Read the model definition and answer for the solid it produces. Units are mm, in the model's axes. A direction names the side the tool comes from. Coordinates: 2 decimals unless noted, no trailing zeros. Write each loop counter-clockwise with the first axis right and the second up, starting at its lowest first coordinate (ties: lowest second). Pieces come first, ordered by that corner, then holes. Notation, with made-up numbers: (86, -5) -> (90, -5) arc R11 ccw to (90, 6) -> close; hole circle Ø7 at (58.5, 63.25). An arc over 180 degrees is marked (long way). Answer in a Markdown table with one row per item. Add a question column.
Item 1: Section B-B on x = 1.25 is taken. Write down the section's boundary in (y, z).
Item 2: Which of the six approach directions +Z, -Z, +X, -X, +Y, -Y give full straight-line access (tool end or side, diameter ignored) to faces 4 (the face through (1, 50, 35.286)), 5 (the face through (-11.25, 22, 6)), 6 (the face through (32.196, -1.479, -2.614)), 7 (the face through (1, 35, 38.286))?
Item 3: Section C-C on y = 48 is taken. Write down the section's boundary in (x, z), then the cut area to 3 significant figures.
Item 4: Given pin 1 Ø10 at (x, y) = (-9, 35) entering from +Z; pin 2 Ø1.5 at (x, z) = (-19.5, 53) entering from +Y; pin 3 Ø12 at (x, z) = (29, 13.5) entering from -Y, each flat-ended and moving along its own axis, determine where each tip first touches the part or whether it passes through.
Item 5: Section D-D on x = 15 is taken. Write down the section's boundary in (y, z), then the cut area to 3 significant figures.
Item 6: Straight lines are drawn through the part: line 1 (Y direction, x = 37, z = 50); line 2 (X direction, y = 31, z = 19.5); line 3 (Y direction, x = 9, z = 26). For each, find the intervals that lie inside material, in ascending order. Write a range as from..to.
Item 7: For a pull along X with two mould halves and no side action, classify faces 1 (the face through (-48.75, 3, 25)), 2 (the face through (-5.8, 19.27, -4.12)), 3 (the face through (13.75, 22, 7)) as +X half, -X half, draft (parallel to the pull), parting line (faces both ways), or undercut.
Item 8: Section A-A on z = 27.5 is taken. Write down the section's boundary in (x, y).
```python
from build123d import *

# Parameters (mm, degrees)
SKETCH1_W           = 100
SKETCH1_H           = 100
BOSS_EXTRUDE1_DEPTH = 38
SKETCH3_R           = 3
BOSS_EXTRUDE2_DEPTH = 3
SKETCH4_R           = 8.25
SKETCH5_R           = 9.5
SKETCH6_W           = 25
SKETCH6_H           = 3
BOSS_EXTRUDE3_DEPTH = 25
CUT_EXTRUDE3_DEPTH  = 32


with BuildPart() as part:
    # Sketch1 → Boss-Extrude1 (new body)
    with BuildSketch(Plane(origin=(0, 0, 0), x_dir=(1, 0, 0), z_dir=(0, 1, 0))):
        with Locations((1.25, -24.285714286)):
            Rectangle(SKETCH1_W, SKETCH1_H)
    extrude(amount=BOSS_EXTRUDE1_DEPTH)

    # Sketch3 → Boss-Extrude2 (add)
    with BuildSketch(Plane.XZ):
        with Locations(Location((-27.034271247, 52.569985533, 0), (0, 0, 90))):
            Circle(SKETCH3_R)
        with Locations(Location((29.534271247, 52.569985533, 0), (0, 0, 90))):
            Circle(SKETCH3_R)
        with Locations(Location((29.534271247, -3.998556962, 0), (0, 0, 90))):
            Circle(SKETCH3_R)
        with Locations(Location((-27.034271247, -3.998556962, 0), (0, 0, 90))):
            Circle(SKETCH3_R)
    extrude(amount=BOSS_EXTRUDE2_DEPTH)

    # Sketch4 → Cut-Loft1 section 0
    with BuildSketch(Plane.XZ):
        with Locations((1.25, 1.285714286)):
            Circle(SKETCH4_R)
    # Sketch5 → Cut-Loft1 section 1
    with BuildSketch(Plane(origin=(0, 38, 0), x_dir=(1, 0, 0), z_dir=(0, 1, 0))):
        with Locations((1.25, -1.285714286)):
            Circle(SKETCH5_R)
    loft(mode=Mode.SUBTRACT)

    # Sketch6 → Boss-Extrude3 (add)
    with BuildSketch(Plane(origin=(0, 38, 0), x_dir=(1, 0, 0), z_dir=(0, 1, 0))):
        with Locations((1.25, -36.785714286)):
            Rectangle(SKETCH6_W, SKETCH6_H)
    extrude(amount=BOSS_EXTRUDE3_DEPTH)

    # Sketch9 → Cut-Extrude3 (cut)
    with BuildSketch(Plane(origin=(0, 38, 0), x_dir=(1, 0, 0), z_dir=(0, 1, 0))):
        Polygon((-49.799740752, 27.751403127), (-11.25, 27.751403127), (-11.25, -38.285714286), (13.75, -38.285714286), (13.75, 28.556619644), (53.406913463, 28.556619644), (53.406913463, -79.342393637), (26.184866917, -79.342393637), (26.184866917, -84.038284162), (-21.600270932, -84.038284162), (-21.600270932, -78.738481249), (-49.799740752, -78.738481249), align=None)
    extrude(amount=-CUT_EXTRUDE3_DEPTH, mode=Mode.SUBTRACT)


solid = part.part
```
Results below:
| question | item | result |
|---|---|---|
| 1 | outline | (0, -25.71) -> (38, -25.71) -> (38, -8.21) -> (0, -6.96) -> close; (0, 9.54) -> (38, 10.79) -> (38, 35.29) -> (63, 35.29) -> (63, 38.29) -> (6, 38.29) -> (6, 74.29) -> (0, 74.29) -> close |
| 2 | face 4 | -Z, +X, -X, +Y |
| 2 | face 5 | +Z, -Z, -X, +Y |
| 2 | face 6 | -Y |
| 2 | face 7 | +Z, +X, -X, +Y |
| 3 | outline | (-11.25, 35.29) -> (13.75, 35.29) -> (13.75, 38.29) -> (-11.25, 38.29) -> close |
| 3 | area | 75.0 mm2 |
| 4 | pin 1 | stops at z = 38.29 |
| 4 | pin 2 | stops at y = 6 |
| 4 | pin 3 | stops at y = 0 |
| 5 | outline | (0, -25.71) -> (6, -25.71) -> (6, 74.29) -> (0, 74.29) -> close |
| 5 | area | 600 mm2 |
| 6 | line 1 | y = 0..6 |
| 6 | line 2 | x = -11.25..13.75 |
| 6 | line 3 | y = 0..38 |
| 7 | face 1 | -X half |
| 7 | face 2 | undercut |
| 7 | face 3 | +X half |
| 8 | outline | (-48.75, 0) -> (51.25, 0) -> (51.25, 6) -> (13.75, 6) -> (13.75, 38) -> (-11.25, 38) -> (-11.25, 6) -> (-48.75, 6) -> close |
